Geometry: see drawing. Coordinates: mm, zero at the bounding-box minimum. Give positions to 0.01 mm unless a question says otherwise; leave off trailing zeros. Order: outer loops, then holes, each group sorted by start corner. A loop starts at its lowest first (then second) coordinate and runs counter-clockwise, first axis right, second up. Notation, with made-up numbers: (-3.75, 52) - (44.25, 52) arc R5 ccw to (44.25, 59) - close; hole circle Ø10 at (22, -4.75). An arc over 180 degrees is marked (long way). Put each result on its own line as item: value. Start each with the question number.
1. Ray query, line 1 along Z through (x, y) = (5, 4.75); line 2 along X through (y, z) = (4, 5). Return the intervals inside material, ascending. Write a range as from..to.
2. Section D-D on x = 22.5. Return the cut outline in (y, z).
3. Section B-B on z = 5. Return the cut outline in (x, y), plus the area to 3 significant figures.
4. First-contact query: P1, Ø3.5, axis at x = 5, z = 21, coming from the -Y side. Flat tip, straight axial feed; report the tip coordinate or a pass-through.
5. Section A-A on y = 1.25. Return the cut outline in (x, z).
6. Section C-C on z = 14.5. Return the cut outline in (x, y), plus the area to 3 significant figures.
7. Mould query, pull axis X, two halves, no side actions, for the marked faces 1, 2 and 3. Classes: pulls with the +X half, pulls with the -X half, needs draft (parallel to the pull), parting line crosses it, or undercut.
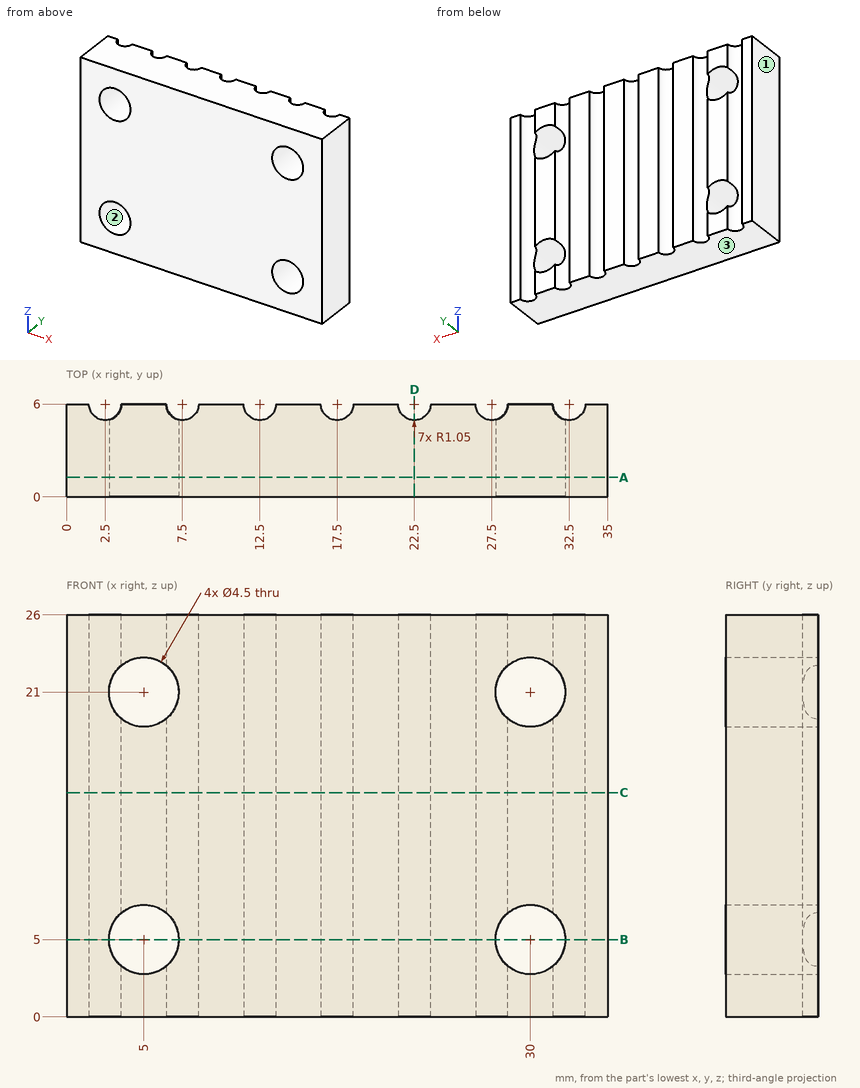
Resolved:
1. line 1: 0..2.75, 7.25..18.75, 23.25..26
1. line 2: 0..2.75, 7.25..27.75, 32.25..35
2. outline: (0, 0) - (4.95, 0) - (4.95, 26) - (0, 26) - close
3. outline: (0, 0) - (2.75, 0) - (2.75, 4.98) arc R1.05 cw to (1.45, 6) - (0, 6) - close; (7.25, 0) - (27.75, 0) - (27.75, 4.98) arc R1.05 cw to (26.45, 6) - (23.55, 6) arc R1.05 cw to (21.45, 6) - (18.55, 6) arc R1.05 cw to (16.45, 6) - (13.55, 6) arc R1.05 cw to (11.45, 6) - (8.55, 6) arc R1.05 cw to (7.25, 4.98) - close; (32.25, 0) - (35, 0) - (35, 6) - (33.55, 6) arc R1.05 cw to (32.25, 4.98) - close
3. area: 146 mm^2
4. P1: through
5. outline: (0, 0) - (35, 0) - (35, 26) - (0, 26) - close; hole circle Ø4.5 at (5, 5); hole circle Ø4.5 at (5, 21); hole circle Ø4.5 at (30, 5); hole circle Ø4.5 at (30, 21)
6. outline: (0, 0) - (35, 0) - (35, 6) - (33.55, 6) arc R1.05 cw to (31.45, 6) - (28.55, 6) arc R1.05 cw to (26.45, 6) - (23.55, 6) arc R1.05 cw to (21.45, 6) - (18.55, 6) arc R1.05 cw to (16.45, 6) - (13.55, 6) arc R1.05 cw to (11.45, 6) - (8.55, 6) arc R1.05 cw to (6.45, 6) - (3.55, 6) arc R1.05 cw to (1.45, 6) - (0, 6) - close
6. area: 198 mm^2
7. face 1: pulls with the -X half
7. face 2: undercut
7. face 3: needs draft
